```python
from build123d import *

# Parameters (mm, degrees)
SKETCH1_W           = 10
SKETCH1_H           = 10
BOSS_EXTRUDE1_DEPTH = 15
SKETCH2_R           = 3.5
CUT_EXTRUDE1_DEPTH  = 1
SKETCH3_R           = 2.65
CUT_EXTRUDE2_DEPTH  = 7.9
SKETCH4_R           = 0.75
CUT_EXTRUDE3_DEPTH  = 21.104974509


with BuildPart() as part:
    # Sketch1 → Boss-Extrude1 (new body)
    with BuildSketch(Plane(origin=(0, 0, 0), x_dir=(1, 0, 0), z_dir=(0, 1, 0))):
        with Locations((5, 5)):
            Rectangle(SKETCH1_W, SKETCH1_H)
    extrude(amount=BOSS_EXTRUDE1_DEPTH)

    # Sketch2 → Cut-Extrude1 (cut)
    with BuildSketch(Plane.XY):
        with Locations((5, 9)):
            Circle(SKETCH2_R)
    extrude(amount=-CUT_EXTRUDE1_DEPTH, mode=Mode.SUBTRACT)

    # Sketch3 → Cut-Extrude2 (cut)
    with BuildSketch(Plane.XY.offset(-1)):
        with Locations((5, 9)):
            Circle(SKETCH3_R)
    extrude(amount=-CUT_EXTRUDE2_DEPTH, mode=Mode.SUBTRACT)

    # Sketch4 → Cut-Extrude3 (cut, through all)
    with BuildSketch(Plane.XY.offset(-8.9)):
        with Locations((5, 9)):
            Circle(SKETCH4_R)
    extrude(amount=-CUT_EXTRUDE3_DEPTH, mode=Mode.SUBTRACT)


solid = part.part
```
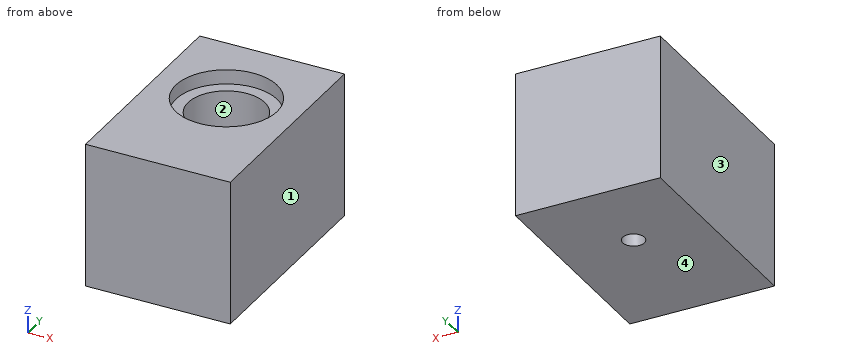
Source: CAD feature listing. Evaluate the final solid. Frame: model axes, mm. Face numbers are marked on the shaded views. Round coordinates to 2 decimals unless told otherwise and drop trailing zeros. Write each loop counter-clockwise with the first axis right and the second up, starting at its lowest first coordinate (ties: lowest second). Pieces come first, ordered by that corner, then holes. Notation, with made-up numbers: M -16,57.5 L 30,57.5 A21 cw 30,91.5 Z; hole C -25,49 d8. An arc over 180 degrees is marked long. Use CSV: the item, a comma, the result in double quotes. Start each with the question number.
Q1. Cut plane B-B on x = 5. Output: boundary loops of the cut face in (y, z).
Q2. First-contact query: P1, Ø2, axis at x = 5, y = 9, coming from the +Z side; P2, Ø4, axis at x = 6, y = 8.5, coming from the +Z side. Flat tips, straight axial feed; report the tip coordinate or a pass-through.
Q3. Pull-direction query (X, two-part tool) for the marked faces 1, 2, 3 and 4; classes: +X half, -X half, draft (parallel to the pull), parting line (faces both ways), or undercut.
Q4. Line query: line 1 (Y direction, x = 5, z = -9.2); line 2 (Y direction, x = 5, z = -0.55); line 3 (X direction, y = 8.75, z = -2). Output: solid intervals per line, ascending. Write a range as from..to.
Q5. Cut plane A-A on y = 9. Output: boundary loops of the cut face in (x, z), plus the area to 3 significant figures.
Q6. Cut plane C-C on z = -8.5. Output: boundary loops of the cut face in (x, y), plus the area to 3 significant figures.
Q7. Cut plane D-D on x = 2.75. Output: boundary loops of the cut face in (y, z).
Results found:
1,outline,"M 0,-10 L 8.25,-10 L 8.25,-8.9 L 6.35,-8.9 L 6.35,-1 L 5.5,-1 L 5.5,0 L 0,0 Z; M 9.75,-10 L 15,-10 L 15,0 L 12.5,0 L 12.5,-1 L 11.65,-1 L 11.65,-8.9 L 9.75,-8.9 Z"
2,P1,"z = -8.9"
2,P2,"z = -1"
3,face 1,"+X half"
3,face 2,"undercut"
3,face 3,"-X half"
3,face 4,"draft"
4,line 1,"0..8.25, 9.75..15"
4,line 2,"0..5.5, 12.5..15"
4,line 3,"0..2.36, 7.64..10"
5,outline,"M 0,-10 L 4.25,-10 L 4.25,-8.9 L 2.35,-8.9 L 2.35,-1 L 1.5,-1 L 1.5,0 L 0,0 Z; M 5.75,-10 L 10,-10 L 10,0 L 8.5,0 L 8.5,-1 L 7.65,-1 L 7.65,-8.9 L 5.75,-8.9 Z"
5,area,"49.5 mm^2"
6,outline,"M 0,0 L 10,0 L 10,15 L 0,15 Z; hole C 5,9 d5.3"
6,area,"128 mm^2"
7,outline,"M 0,-10 L 15,-10 L 15,0 L 11.68,0 L 11.68,-1 L 10.4,-1 L 10.4,-8.9 L 7.6,-8.9 L 7.6,-1 L 6.32,-1 L 6.32,0 L 0,0 Z"
